Autodesk Inventor part; units mm, degrees
ref_plane "Work Plane1" through (-8.1417, 0, 0) normal (0, -0.866, -0.5) x (1, 0, 0)
ref_plane "YZ Plane" through (0, 0, 0) normal (1, 0, 0) x (0, 1, 0)
ref_plane "XZ Plane" through (0, 0, 0) normal (0, 1, 0) x (-1, 0, 0)
sketch "Sketch1" plane through (0, 0, 0) normal (1, 0, 0) x (0, 1, 0)
  line L0 (-4.6188, 0) -> (-2.3094, 4)
  line L1 (-2.3094, 4) -> (2.3094, 4)
  line L2 (2.3094, 4) -> (4.6188, 0)
  line L3 (4.6188, 0) -> (2.3094, -4)
  line L4 (2.3094, -4) -> (-2.3094, -4)
  line L5 (-2.3094, -4) -> (-4.6188, 0)
  point P0 (0, 0)
  point P1 (0, 0)
  dimension "d0" = 9.2376
extrude "Body" add sketch "Sketch1" along normal blind 5.1
sketch "Sketch2" plane through (0, 0, 0) normal (0, 0, 1) x (1, 0, 0)
  line L0 (0, 2.3094) -> (0, 4.6188)
  line L1 (0, 4.6188) -> (5.1, 4.6188)
  line L2 (5.1, 2.3094) -> (5.1, 4.6188)
  line L3 (-1.02, 0) -> (6.12, 0)
  line L4 (0.3573, 4.6188) -> (0, 4)
  line L5 (4.7427, 4.6188) -> (5.1, 4)
  dimension "d3" = 30
  dimension "d4" = 30
  dimension "d5" = 8
  dimension "d6" = 8
revolve "Chamfer1" cut sketch "Sketch2" angle 360 about axis through (-10, 0, 0) along (1, 0, 0)
sketch "Sketch3" plane through (5.1, 0, 0) normal (1, 0, 0) x (0, 0, -1)
  arc A0 (-2, -3.4641) -> (2, -3.4641) centre (0, 0) ccw
hole "Thread" at (5.1, 0, 0) direction (-1, 0, 0) diameter 4.134 end through all
chamfer "Chamfer2" distance 0.433 angle 30 1 edges at (5.1, 0, 2.067) measured on face at (5.1, 3.336, -0.083)
chamfer "Chamfer3" distance 0.433 angle 30 1 edges at (0, 0, 2.067) measured on face at (0, 3.336, -0.083)
ref_plane "Work Plane1" through (-8.1417, 0, 0) normal (0, -0.866, -0.5) x (1, 0, 0)
equation "\"d0\" = 1.1547 * SW"
equation "\"d1\" = KOH"
equation "\"d3\" = ANG1"
equation "\"d4\" = ANG2"
equation "\"d5\" = SW0"
equation "\"d6\" = SW01"
equation "\"d8\" = -0.5 * GD1 + 0.5 * NND"
equation "\"d40\" = -0.5 * GD1 + 0.5 * NND"
equation "\"d10\" = -0.5 * GD1 + 0.5 * NND"
equation "\"d41\" = -0.5 * GD1 + 0.5 * NND"
equation "\"ANG1\" = 30deg"
equation "\"ANG2\" = 30deg"
equation "\"NND\" = 5"
equation "\"KOH\" = 5.1"
equation "\"SW\" = 8"
equation "\"SW0\" = SW"
equation "\"SW01\" = SW"
equation "\"GUL\" = 0.541266 * PTC"
equation "\"THREADDIA\" = 5"
equation "\"TOA\" = 30deg"
equation "\"PTC\" = 0.8"
equation "\"E0\" = 1.155 * SW"
equation "\"GAL\" = 0.541266 * PTC"
equation "\"SD2\" = 0"
equation "\"WFT\" = 0"
properties part number "ANSI B18.2.4.2M - M5 x 0.8" material "Steel, Mild"
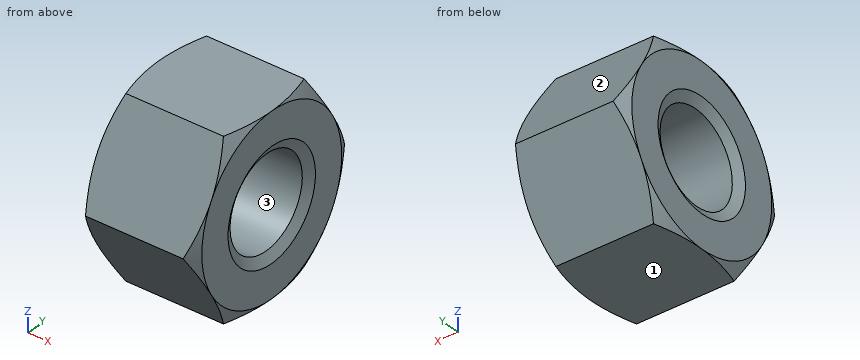
The listing builds one solid part. Answer for the finished solid, in the listing's coordinates (mm). Face numbers are marked on the shaded views. Round coordinates to 2 decimals unless told otherwise and drop trailing zeros. Write each loop counter-clockwise with the first axis right and the second up, starting at its lowest first coordinate (ties: lowest second). Pieces come first, ordered by that corner, then holes. Notation, with made-up numbers: (6.5, -17.75) - (62.5, -17.75) arc R12 cw to (62.5, -8.75) - close; hole circle Ø2 at (45, 48.25). An arc over 180 degrees is marked (long way). Use a Markdown table: item, result. Add a question column.
1. For a pull along Y with two mould halves and no side action, classify the marked faces 1, 2 and 3 as +Y half, -Y half, draft (parallel to the pull), parting line (faces both ways), or undercut.
2. Consider line 1 (Z direction, x = 0.7, y = 0); line 2 (Y direction, x = 1.45, z = -0.5); line 3 (Z direction, x = 2.8, y = -1.5). Determine where each line is inside the solid, lowest interval first.
3. The part is cut by section A-A (x = 2.25). Write down the section's boundary in (y, z).
4. Flat-ended cylindrical pins translate along their axes: P1, Ø2, axis at x = 3, z = 2.5, coming from the +Y side; P2, Ø1.5, axis at y = -2, z = 0, coming from the +X side. Find the tip coordinate at first contact, or state that the pin passes through.
Reported:
| question | item | result |
|---|---|---|
| 1 | face 1 | draft |
| 1 | face 2 | +Y half |
| 1 | face 3 | undercut |
| 2 | line 1 | -4 to -2.07, 2.07 to 4 |
| 2 | line 2 | -4.33 to -2.01, 2.01 to 4.33 |
| 2 | line 3 | -4 to -1.42, 1.42 to 4 |
| 3 | outline | (-4.62, 0) - (-2.31, -4) - (2.31, -4) - (4.62, 0) - (2.31, 4) - (-2.31, 4) - close; hole circle Ø4.13 at (0, 0) |
| 4 | P1 | y = 3.75 |
| 4 | P2 | x = 5.1 |
